```python
from build123d import *

# Parameters (mm, degrees)
F0_W      = 152.4
F0_H      = 304.8
F1_DEPTH  = 5.08
F2_W      = 152.4
F2_H      = 304.8
F2_W_2    = 142.2399785995
F2_H_2    = 294.6399785995
F3_DEPTH  = 25.4
F4_W      = 152.4
F4_H      = 304.8
F4_W_2    = 142.2399785995
F4_H_2    = 294.6399785995
F4_W_3    = 128.0160005927
F4_H_3    = 280.4160005927
F5_DEPTH  = 5.08
F6_R      = 12.7
F7_W      = 32.2413705289
F7_H      = 15.166670084
F8_DEPTH  = 25.4
F9_R      = 5.07999
F10_W     = 24.1091474891
F10_H     = 8.1412196159
F11_DEPTH = 25.4


# Not quite as in the source:
# - a fillet or chamfer is up to 0.001 mm smaller than in the source, because OpenCascade refuses the exact size


with BuildPart() as f1:
    # F0 (on Top) → F1 (new body)
    with BuildSketch(Plane.XY):
        with Locations((-76.2, 152.4)):
            Rectangle(F0_W, F0_H)
    extrude(amount=F1_DEPTH)

    # F2 (on face) → F3 (join)
    with BuildSketch(Plane.XY.offset(5.08)):
        with Locations((-76.2, 152.4)):
            Rectangle(F2_W, F2_H)
        with Locations((-76.2, 152.4)):
            Rectangle(F2_W_2, F2_H_2, mode=Mode.SUBTRACT)
    extrude(amount=F3_DEPTH)

    # F4 (on face) → F5 (join)
    with BuildSketch(Plane.XY.offset(30.48)):
        with Locations((-76.2, 152.4)):
            Rectangle(F4_W, F4_H)
        with Locations((-76.2, 152.4)):
            Rectangle(F4_W_2, F4_H_2, mode=Mode.SUBTRACT)
        with Locations((-76.2, 152.4)):
            Rectangle(F4_W_2, F4_H_2)
        with Locations((-76.2, 152.4)):
            Rectangle(F4_W_3, F4_H_3, mode=Mode.SUBTRACT)
    extrude(amount=F5_DEPTH)

    # F6
    f6_edges = [f1.edges().sort_by_distance(p)[0] for p in [
        (-152.4, 0, 17.78),
        (0, 0, 17.78),
        (0, 304.8, 17.78),
        (-152.4, 304.8, 17.78),
        (-147.319989, 5.080011, 17.78),
        (-5.080011, 5.080011, 17.78),
        (-5.080011, 299.719989, 17.78),
        (-147.319989, 299.719989, 17.78),
        (-140.208, 12.192, 33.02),
        (-12.192, 292.608, 33.02),
        (-140.208, 292.608, 33.02),
        (-12.192, 12.192, 33.02),
    ]]
    fillet(f6_edges, radius=F6_R)

    # F7 (on face) → F8 (cut)
    with BuildSketch(Plane(origin=(0, 0, 0), x_dir=(1, 0, 0), z_dir=(0, 0, -1))):
        with Locations((-35.8565431088, -276.2855738401)):
            Rectangle(F7_W, F7_H)
    extrude(amount=-F8_DEPTH, mode=Mode.SUBTRACT)

    # F9 (radius 5.08 in the source; OpenCascade refuses exactly that, so slightly less here)
    f9_edges = [f1.edges().sort_by_distance(p)[0] for p in [
        (-51.977228, 283.868909, 2.54),
        (-19.735858, 283.868909, 2.54),
        (-19.735858, 268.702239, 2.54),
        (-51.977228, 268.702239, 2.54),
        (-76.2, 304.8, 35.56),
        (-3.719744, 301.080256, 35.56),
        (-148.680256, 301.080256, 35.56),
        (0, 152.4, 35.56),
        (-152.4, 152.4, 35.56),
        (-3.719744, 3.719744, 35.56),
        (-148.680256, 3.719744, 35.56),
        (-76.2, 0, 35.56),
        (-140.208, 152.4, 35.56),
        (-136.488256, 15.911744, 35.56),
        (-136.488256, 288.888256, 35.56),
        (-76.2, 12.192, 35.56),
        (-76.2, 292.608, 35.56),
        (-15.911744, 15.911744, 35.56),
        (-15.911744, 288.888256, 35.56),
        (-12.192, 152.4, 35.56),
    ]]
    fillet(f9_edges, radius=F9_R)

    # F10 (on face) → F11 (cut)
    with BuildSketch(Plane(origin=(0, 0, 0), x_dir=(1, 0, 0), z_dir=(0, 0, -1))):
        with Locations((-110.6483452022, -273.3389437199)):
            Rectangle(F10_W, F10_H)
    extrude(amount=-F11_DEPTH, mode=Mode.SUBTRACT)


solid = f1.part
```
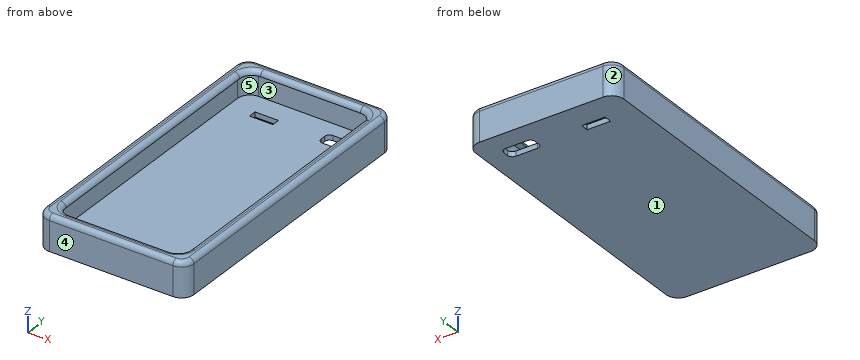
Geometry: final body of the model. Coordinates: model frame, mm. Face numbers are marked on the shaded views. A direction names the side the tool comes from. Round coordinates to 2 decimals unless told otherwise and drop trailing zeros. Write each loop counter-clockwise with the first axis right and the second up, starting at its lowest first coordinate (ties: lowest second). Pieces come first, ordered by that corner, then holes. Notation, with made-up numbers: (31.25, 32.25) -> (61.25, 32.25) arc R13 ccw to (61.25, 43.25) -> close; hole circle Ø2 at (14, 30.5). An arc over 180 degrees is marked (long way). Use CSV: the item, a comma, the result in double quotes. Start each with the question number.
Q1. Reachability of the marked faces 4 and 5 from +Z, -Z, +X, -X, +Y, -Y: full face, straight path, thin tool, end or side. Return the list, or none.
Q2. Section B-B (z = 21). Return loops of the section in (x, y).
Q3. Pull-direction query (Z, two-part tool) for the marked faces 1, 2 and 3; classes: pulls with the +Z half, pulls with the -Z half, needs draft (parallel to the pull), parting line crosses it, or undercut.
Q4. First-contact query: pin 1 Ø6 at (x, y) = (-119.5, 242.5) entering from +Z; pin 2 Ø4 at (x, y) = (-82.5, 252) entering from -Z. Flat tips, straight axial feed; report the tip coordinate or a pass-through.
Q5. Line query: L1, parallel to Y at x = -117, z = 29; L2, parallel to X at y = 279.5, z = 11.5; L3, parallel to Y at x = -15.5, z = 24. Output: solid intervals per line, ascending.
Result sheet:
1,face 4,"+Z, -Z, +X, -X, -Y"
1,face 5,"none"
2,outline,"(-152.4, 12.7) arc R12.7 ccw to (-139.7, 0) -> (-12.7, 0) arc R12.7 ccw to (0, 12.7) -> (0, 292.1) arc R12.7 ccw to (-12.7, 304.8) -> (-139.7, 304.8) arc R12.7 ccw to (-152.4, 292.1) -> close; hole (-147.32, 17.78) arc R12.7 ccw to (-134.62, 5.08) -> (-17.78, 5.08) arc R12.7 ccw to (-5.08, 17.78) -> (-5.08, 287.02) arc R12.7 ccw to (-17.78, 299.72) -> (-134.62, 299.72) arc R12.7 ccw to (-147.32, 287.02) -> close"
3,face 1,"pulls with the -Z half"
3,face 2,"needs draft"
3,face 3,"undercut"
4,pin 1,"z = 5.08"
4,pin 2,"z = 0"
5,L1,"0 to 5.08, 299.72 to 304.8"
5,L2,"-152.4 to -147.32, -5.08 to 0"
5,L3,"0 to 5.29, 299.51 to 304.8"
